Can you work these out from the model? Positions are in its coordinate system, mm. Face numbers are marked on the shaded views. A direction names the side the tool comes from. Give positions to 0.01 mm unless a question says otherwise; leave off trailing zeros. Order: outer loops, then holes, each group sorted by start corner. A loop starts at its lowest first (then second) coordinate and runs counter-clockwise, first axis right, second up. Notation, with made-up numbers: (-22.75, 26.25) - (-16.75, 26.25) arc R30 cw to (-16.75, 54.25) - close; hole circle Ø4 at (79, 11.5). An arc over 180 degrees is marked (long way). Answer as a JSON object with one key per item and string values.
```python
from build123d import *

# Parameters (mm, degrees)
EXTRUDE_1_DEPTH       = 68
SKETCH_2_R            = 1.5
CUT_EXTRUDE_1_DEPTH   = 60
SKETCH_3_W            = 30
SKETCH_3_H            = 4
EXTRUDE_2_DEPTH       = 40
EXTRUDE_3_DEPTH       = 30
CUT_EXTRUDE_2_DEPTH   = 4
EXTRUDE_4_DEPTH       = 23
EXTRUDE_START         = -53
EXTRUDE_5_DEPTH       = 23
EXTRUDE_6_DEPTH       = 3
EXTRUDE_7_DEPTH       = 0.66666
SKETCH_17_W           = 17.087989765
SKETCH_17_H           = 19.996406133
EXTRUDE_9_DEPTH       = 12
SKETCH_19_R           = 1.8
CUT_EXTRUDE_3_DEPTH   = 20
SKETCH_20_W           = 61.603006609
SKETCH_20_H           = 84.586869481
CUT_EXTRUDE_4_DEPTH   = 65
SKETCH_21_W           = 7.494214953
SKETCH_21_H           = 26.873102225
CUT_EXTRUDE_5_DEPTH   = 2
SKETCH_22_W           = 9.970658679
SKETCH_22_H           = 25.794738871
CUT_EXTRUDE_6_DEPTH   = 2
EXTRUDE_10_DEPTH      = 4
EXTRUDE_11_DEPTH      = 12
EXTRUDE_11_DEPTH_BACK = 12


with BuildPart() as part:
    # 草图1 → 凸台-拉伸1 (new body)
    with BuildSketch(Plane(origin=(0, 0, 0), x_dir=(0, 0, -1), z_dir=(1, 0, 0))):
        Polygon((0, 0), (0, 4), (-10, 4), (-10, 7), (0, 7), (0, 10), (-14, 10), (-14, 0), align=None)
    extrude(amount=EXTRUDE_1_DEPTH)

    # 草图2 → 切除-拉伸1 (cut)
    with BuildSketch(Plane(origin=(0, 10, 0), x_dir=(1, 0, 0), z_dir=(0, 1, 0))):
        with Locations(Location((5, -3.5, 0), (0, 0, 270))):
            Circle(SKETCH_2_R)
        with Locations(Location((63, -3.5, 0), (0, 0, 270))):
            Circle(SKETCH_2_R)
    extrude(amount=-CUT_EXTRUDE_1_DEPTH, mode=Mode.SUBTRACT)

    # 草图3 → 凸台-拉伸2 (add)
    with BuildSketch(Plane.XZ):
        with Locations((34, 12)):
            Rectangle(SKETCH_3_W, SKETCH_3_H)
    extrude(amount=-EXTRUDE_2_DEPTH)

    # 草图4 → 凸台-拉伸3 (add)
    with BuildSketch(Plane(origin=(49, 0, 0), x_dir=(0, 0, -1), z_dir=(1, 0, 0))):
        Polygon((-14, 40), (-26.357684131, 54.727314459), (-23.293506358, 57.298464898), (-10, 41.455880937), (-10, 40), align=None)
    extrude(amount=-EXTRUDE_3_DEPTH)

    # 草图5 → 切除-拉伸2 (cut)
    with BuildSketch(Plane(origin=(0, 9.633382176, -11.480617817), x_dir=(1, 0, 0), z_dir=(0, -0.6427876096865429, 0.7660444431189751))):
        with BuildLine():
            Line((25.25, 55.318123989), (25.25, 43.864814933))
            ThreePointArc((25.25, 43.864814933), (23.75, 42.364814933), (22.25, 43.864814933))
            Line((22.25, 43.864814933), (22.25, 55.318123989))
            ThreePointArc((22.25, 55.318123989), (23.75, 56.818123989), (25.25, 55.318123989))
        make_face()
        with BuildLine():
            Line((42.75, 55.318123989), (42.75, 43.864814933))
            ThreePointArc((42.75, 43.864814933), (44.25, 42.364814933), (45.75, 43.864814933))
            Line((45.75, 43.864814933), (45.75, 55.318123989))
            ThreePointArc((45.75, 55.318123989), (44.25, 56.818123989), (42.75, 55.318123989))
        make_face()
    extrude(amount=-CUT_EXTRUDE_2_DEPTH, mode=Mode.SUBTRACT)

    # 草图6 → 凸台-拉伸4 (add)
    with BuildSketch(Plane.ZY.offset(-19)):
        Polygon((23.293506358, 57.298464898), (26.357684131, 54.727314459), (14, 40), (10.935822228, 42.571150439), align=None)
    extrude(amount=EXTRUDE_4_DEPTH)

    # 草图7 → 凸台-拉伸5 (add)
    with BuildSketch(Plane.ZY.offset(4).offset(EXTRUDE_START)):
        Polygon((23.293506358, 57.298464898), (26.357684131, 54.727314459), (14, 40), (10.935822228, 42.571150439), align=None)
    extrude(amount=-EXTRUDE_5_DEPTH)

    # 草图10 → 凸台-拉伸6 (add)
    with BuildSketch(Plane(origin=(52, 0, 0), x_dir=(0, 0.7660444431189749, 0.6427876096865431), z_dir=(-1, 0, 0))):
        Polygon((39.64080426, 18.986882184), (58.865947907, 18.986882184), (58.865947907, 25.653542184), (39.64080426, 20.653542184), align=None)
    extrude(amount=-EXTRUDE_6_DEPTH)

    # 草图15 → 凸台-拉伸7 (add)
    with BuildSketch(Plane(origin=(-0.224740323, 0.898508111, -2.01476807), x_dir=(0.9948507831271028, 0.04127952147527669, -0.09256306184522162), z_dir=(0.10135047760810084, -0.4051975406133526, 0.9085939873064868))):
        Polygon((55.510576319, 63.468125115), (55.510576319, 62.353864223), (55.510576319, 43.471718982), (72.598566084, 43.471718982), (72.598566084, 62.353864223), (72.598566084, 63.468125115), align=None)
    extrude(amount=-EXTRUDE_7_DEPTH)

    # 草图17 → 凸台-拉伸9 (add)
    with BuildSketch(Plane(origin=(-0.224740323, 0.898508111, -2.01476807), x_dir=(0.994850783127103, 0.04127952147527699, -0.09256306184522194), z_dir=(0.10135047760810126, -0.40519754061335256, 0.9085939873064869))):
        with Locations((64.054571201, 53.469922049)):
            Rectangle(SKETCH_17_W, SKETCH_17_H)
    extrude(amount=EXTRUDE_9_DEPTH)

    # 草图19 → 切除-拉伸3 (cut)
    with BuildSketch(Plane(origin=(-0.292306632, 1.168637103, -2.620491338), x_dir=(-0.9948507831271028, -0.04127952147527692, 0.09256306184522202), z_dir=(-0.10135047760810131, 0.40519754061335245, -0.908593987306487))):
        with Locations(Location((-62.598566084, 60.969922048, 0), (0, 0, 90))):
            Circle(SKETCH_19_R)
        with Locations(Location((-62.598566084, 45.969922048, 0), (0, 0, 270))):
            Circle(SKETCH_19_R)
    extrude(amount=-CUT_EXTRUDE_3_DEPTH, mode=Mode.SUBTRACT)

    # 草图20 → 切除-拉伸4 (cut)
    with BuildSketch(Plane.ZY.offset(-34)):
        with Locations((16.944749698, 32.191708304)):
            Rectangle(SKETCH_20_W, SKETCH_20_H)
    extrude(amount=CUT_EXTRUDE_4_DEPTH, mode=Mode.SUBTRACT)

    # 镜向7: part across plane


with BuildPart() as part_1:
    add(part.part)
    add(part.part.mirror(Plane.ZY.offset(-34)))

    # 草图21 → 切除-拉伸5 (cut)
    with BuildSketch(Plane(origin=(-0.292306632, 1.168637103, -2.620491338), x_dir=(-0.9948507831271028, -0.04127952147527692, 0.09256306184522202), z_dir=(-0.10135047760810131, 0.40519754061335245, -0.908593987306487))):
        with Locations((-54.514442647, 53.802326892)):
            Rectangle(SKETCH_21_W, SKETCH_21_H)
    extrude(amount=CUT_EXTRUDE_5_DEPTH, mode=Mode.SUBTRACT)

    # 草图22 → 切除-拉伸6 (cut)
    with BuildSketch(Plane(origin=(0.990797146, 3.961190673, -8.882368888), x_dir=(-0.9948507831271028, 0.04127952147527693, -0.09256306184522203), z_dir=(0.10135047760810131, 0.40519754061335256, -0.9085939873064868))):
        with Locations((-12.026553315, 54.032339334)):
            Rectangle(SKETCH_22_W, SKETCH_22_H)
    extrude(amount=CUT_EXTRUDE_6_DEPTH, mode=Mode.SUBTRACT)

    # 草图24 → 凸台-拉伸10 (add)
    with BuildSketch(Plane.XY.offset(14)):
        Polygon((19, 40), (3.059166743, 10), (8.395226669, 10), (19, 29.957752195), align=None)
        Polygon((49, 40), (64.940833257, 10), (59.604773331, 10), (49, 29.957752195), align=None)
    extrude(amount=-EXTRUDE_10_DEPTH)

    # 草图29 → 凸台-拉伸11 (add, two sides: drawn at the far end of the back side and taken through both)
    with BuildSketch(Plane.ZY.offset(-34).offset(-EXTRUDE_11_DEPTH_BACK)):
        Polygon((10, 10), (2.792361366, 10), (10, 41.455880937), align=None)
    extrude(amount=EXTRUDE_11_DEPTH + EXTRUDE_11_DEPTH_BACK)


solid = part_1.part
```
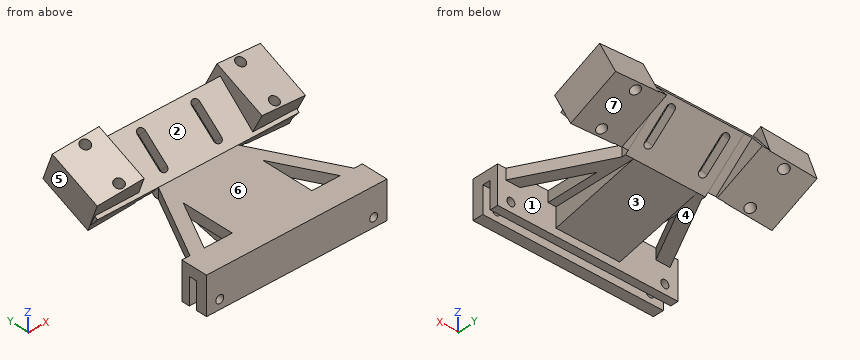
Q1. If we section it at B-B, the plane x = 40.5: Please give me the cut outline in (y, z), then the cut area to 3 significant figures.
Recorded:
{"outline": "(0, 0) - (4, 0) - (4, 10) - (7, 10) - (7, 0) - (10, 0) - (10, 2.79) - (41.46, 10) - (57.3, 23.29) - (54.73, 26.36) - (40, 14) - (0, 14) - close", "area": "426 mm^2"}
Q2. I need wall thicknesses on L1, parallel to X at y = 8.3, z = 3.5; L2, parallel to X at y = 40.5, z = 18; L3, parallel to X at y = 11.5, z = 13.5. Which ranges of each line are inside material? Lowest first, please.
Recorded:
{"L1": "x = 0 to 3.5, 6.5 to 61.5, 64.5 to 68", "L2": "x = -4.97 to 4.36, 5.81 to 12.21, 55.79 to 62.19, 63.64 to 72.97", "L3": "x = 3.86 to 9.19, 19 to 49, 58.81 to 64.14"}
Q3. If we section it at C-C, the plane y = 27.5: Please give me the cut outline in (x, z).
Recorded:
{"outline": "(12.36, 10) - (17.69, 10) - (17.69, 14) - (12.36, 14) - close; (19, 10) - (22, 10) - (22, 6.8) - (46, 6.8) - (46, 10) - (49, 10) - (49, 14) - (19, 14) - close; (50.31, 10) - (55.64, 10) - (55.64, 14) - (50.31, 14) - close"}
Q4. We'd pull the mould along Y, two halves only. Please class the marked faces 1, 2, 3 and 4: released by +Y, released by -Y, zero draft, split by the parting line, or undercut.
Recorded:
{"face 1": "undercut", "face 2": "released by -Y", "face 3": "released by +Y", "face 4": "undercut"}
Q5. If we section it at A-A, the plane y = 12.5: Please give me the cut outline in (x, z), then the cut area to 3 significant figures.
Recorded:
{"outline": "(4.39, 10) - (9.72, 10) - (9.72, 14) - (4.39, 14) - close; (19, 10) - (22, 10) - (22, 3.37) - (46, 3.37) - (46, 10) - (49, 10) - (49, 14) - (19, 14) - close; (58.28, 10) - (63.61, 10) - (63.61, 14) - (58.28, 14) - close", "area": "322 mm^2"}
Q6. Which directions (+Z, -Z, +X, -X, +Y, -Y) give clear straight access to the entire face, cutting with the end or side of a thin tool? Please do the marked faces 5, 6 and 7.
Recorded:
{"face 5": "-Z, -X, +Y", "face 6": "+Z, +X, -X, -Y", "face 7": "-Z, +Y"}
Q7. I'm going to push flat-ended pins straight in: pin 1 Ø8 at (x, y) = (50.5, 35) entering from +Z; pin 2 Ø0.8 at (y, z) = (41.5, 12.5) entering from +X; pin 3 Ø1.2 at (y, z) = (17, 11) entering from -X; pin 4 Ø1.8 at (x, z) = (63, 3.5) entering from +Y. Where does each tip first touch, or does it pass through?
Recorded:
{"pin 1": "stops at z = 14", "pin 2": "stops at x = 72", "pin 3": "stops at x = 6.46", "pin 4": "passes through"}
